```python
from build123d import *

# Parameters (mm, degrees)
SKETCH1_R           = 2
BOSS_EXTRUDE1_DEPTH = 5
SKETCH2_W           = 18
SKETCH2_H           = 1
CUT_EXTRUDE1_DEPTH  = 6
LPATTERN1_COUNT     = 5
LPATTERN1_PITCH     = 4
LPATTERN1_COL_COUNT = 6
LPATTERN1_COL_PITCH = 4


with BuildPart() as part:
    # Sketch1 → Boss-Extrude1 (new body)
    with BuildSketch(Plane(origin=(0, 0, 0), x_dir=(1, 0, 0), z_dir=(0, 1, 0))):
        with BuildLine():
            Line((5, 41.5), (5, -41.5))
            ThreePointArc((5, -41.5), (0, -46.5), (-5, -41.5))
            Line((-5, -41.5), (-5, 41.5))
            ThreePointArc((-5, 41.5), (0, 46.5), (5, 41.5))
        make_face()
        with Locations((0, 41.5)):
            Circle(SKETCH1_R, mode=Mode.SUBTRACT)
        with Locations((0, -41.5)):
            Circle(SKETCH1_R, mode=Mode.SUBTRACT)
    extrude(amount=BOSS_EXTRUDE1_DEPTH)

    # Sketch2 → Cut-Extrude1 (cut, through all)
    with BuildSketch(Plane(origin=(0, 5, 0), x_dir=(1, 0, 0), z_dir=(0, 1, 0))):
        with Locations((5, 3)):
            Rectangle(SKETCH2_W, SKETCH2_H)
        with Locations((-5, 1)):
            Rectangle(SKETCH2_W, SKETCH2_H)
    cut_extrude1 = extrude(amount=-CUT_EXTRUDE1_DEPTH, mode=Mode.SUBTRACT)

    # LPattern1: Cut-Extrude1 ×5
    with Locations(*[(0, 0, -i * LPATTERN1_PITCH) for i in range(1, LPATTERN1_COUNT)]):
        add(cut_extrude1, mode=Mode.SUBTRACT)

    # LPattern1 col: Cut-Extrude1 ×6
    with Locations(*[(0, 0, i * LPATTERN1_COL_PITCH) for i in range(1, LPATTERN1_COL_COUNT)]):
        add(cut_extrude1, mode=Mode.SUBTRACT)


solid = part.part
```
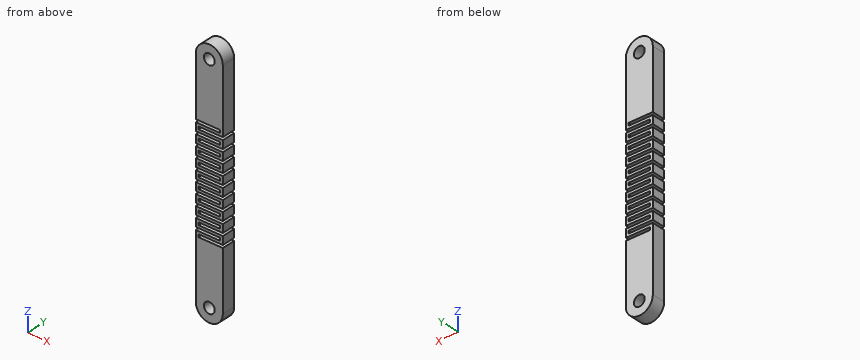
Build history of the part. All positions in model axes, mm. Round coordinates to 2 decimals unless told otherwise and drop trailing zeros.
1) Band-saw the part on A-A, the plane x = -3. Give the number of separate pieces and of enclosed holes in the cut face, and give its area (3 significant figures).
2) Pin check, flat tips, straight feed: pin 1 (2.5 mm diameter, centred on x = 2, y = 2.5, fed in from +Z); pin 2 (1.5 mm diameter, centred on x = -1, y = 3.5, fed in from -Z); pin 3 (0.5 mm diameter, centred on y = 2, z = 13, fed in from +X). Stop position of each tip, or through.
3) Drill centre line: probe 1 along X at (y, z) = (4, -41.5). Where is it in solid material? Low to high.
Ans:
1. separate pieces: 21
1. enclosed holes: 0
1. area: 355 mm2
2. pin 1: stops at z = 46.44
2. pin 2: stops at z = -46.49
2. pin 3: stops at x = -4
3. probe 1: x = -5 to -2, 2 to 5
